from build123d import *

# Parameters (mm, degrees)
EXTRUDE_THIN1_DEPTH = 206.375
FILLET1_R           = 1.27


with BuildPart() as part:
    # Sketch1 → Extrude-Thin1 (new body)
    with BuildSketch(Plane.XY):
        with BuildLine():
            Line((0, 0), (-1.5875, 0))
            Line((-1.5875, 0), (-1.5875, 2.38125))
            ThreePointArc((-1.5875, 2.38125), (-4.95373921, 4.191798454), (-6.35, 7.749902995))
            ThreePointArc((-6.35, 7.749902995), (-7.0533091, 9.486054835), (-8.73125, 10.31875))
            Line((-8.73125, 10.31875), (-8.73125, 11.90625))
            ThreePointArc((-8.73125, 11.90625), (-10.983204711, 13.93861616), (-10.254760064, 16.883303007))
            ThreePointArc((-10.254760064, 16.883303007), (-8.456232552, 18.243920166), (-6.35, 19.05))
            Line((-6.35, 19.05), (-6.35, 20.6375))
            Line((-6.35, 20.6375), (0, 20.6375))
            Line((0, 20.6375), (0, 19.3675))
            Line((0, 19.3675), (-5.08, 19.3675))
            Line((-5.08, 19.3675), (-5.08, 17.961479369))
            ThreePointArc((-5.08, 17.961479369), (-7.394462244, 17.359516713), (-9.353746016, 15.988275809))
            ThreePointArc((-9.353746016, 15.988275809), (-9.540424793, 13.84093001), (-7.46125, 13.272621004))
            Line((-7.46125, 13.272621004), (-7.46125, 11.290352642))
            ThreePointArc((-7.46125, 11.290352642), (-5.752972349, 9.885293584), (-5.080314797, 7.778178184))
            ThreePointArc((-5.080314797, 7.778178184), (-3.615692697, 4.649806034), (-0.3175, 3.623280274))
            Line((-0.3175, 3.623280274), (-0.3175, 1.27))
            Line((-0.3175, 1.27), (0, 1.27))
            Line((0, 1.27), (0, 0))
        make_face()
    extrude(amount=-EXTRUDE_THIN1_DEPTH)

    # Fillet1
    fillet1_edges = [part.edges().sort_by_distance(p)[0] for p in [
        (-5.08, 17.961479369, -103.1875),
        (-7.46125, 13.272621004, -103.1875),
        (-6.35, 20.6375, -103.1875),
    ]]
    fillet(fillet1_edges, radius=FILLET1_R)


solid = part.part
Check sheet for the modelled part. Datum: model origin and axes. Units: mm. A direction names the side the tool comes from. Give positions to 0.01 mm unless a question says otherwise; leave off trailing zeros. Loops run counter-clockwise (first coordinate to the right, second up) from the corner with the lowest first, then second, coordinate; pieces in that order, holes last. Notation, with made-up numbers: M 69.5,71 L 81.5,71 A30 cw 81.5,104 Z; hole C 12,28 d8. An arc over 180 degrees is marked long. Use a Markdown table: item, result. Add a question column.
Q1. Scan lines: line 1 along Y through (x, z) = (-4.75, -111); line 2 along Y through (x, z) = (-0.5, -190.5); line 3 along X through (y, z) = (7.5, -77). Record each from-to range of solid material in increasing order. Write a range as [from, to].
Q2. Sectioned sample at B-B, the plane x = -3.25. Record the cut outline in (y, z) (1 decimal).
Q3. Go/stop test with flat-tipped pins: pin 1 (1.2 mm diameter, centred on y = 1, z = -84.5, fed in from -X); pin 2 (6 mm diameter, centred on y = 9.5, z = -105, fed in from -X); pin 3 (1 mm diameter, centred on y = 9.5, z = -44.5, fed in from +X). Record where each tip stops, or that it passes through.
Q4. Mould release check, pull along Y, two halves, no side actions. Record for faces 1 (the cylindrical face through (-7.817, 17.146, -101.743)), 2 (the flat face through (-6.4, 10.4, -206.375)), 3 (the cylindrical face through (-11, 14, -102)), 4 (the flat face through (-3, 20.638, -102)): pulls with the +Y half, pulls with the -Y half, needs draft (parallel to the pull), parting line crosses it, or undercut.
Q5. Tool access check on faces 5 (the cylindrical face through (-8.48, 18.23, -101.74)), 6 (the flat face through (-3, 19.368, -102)). Record the directions out of +Z, -Z, +X, -X, +Y, -Y that give a thin tool (end or side, any length) a straight path to the whole face; none if there is none.
Q6. Sectioned sample at A-A, the plane z = -132. Record the cut outline in (x, y), then the cut area to 3 significant figures.
Verdict:
| question | item | result |
|---|---|---|
| 1 | line 1 | [3.97, 6.22], [19.37, 20.64] |
| 1 | line 2 | [0, 3.61], [19.37, 20.64] |
| 1 | line 3 | [-6.34, -5.07] |
| 2 | outline | M 2.9,-206.4 L 4.4,-206.4 L 4.4,0 L 2.9,0 Z; M 19.4,-206.4 L 20.6,-206.4 L 20.6,0 L 19.4,0 Z |
| 3 | pin 1 | x = -1.59 |
| 3 | pin 2 | x = -10.01 |
| 3 | pin 3 | x = -5.3 |
| 4 | face 1 | undercut |
| 4 | face 2 | needs draft |
| 4 | face 3 | parting line crosses it |
| 4 | face 4 | pulls with the +Y half |
| 5 | face 5 | +Z, -Z, -X, +Y |
| 5 | face 6 | +Z, -Z, +X |
| 6 | outline | M -10.25,16.88 A2.95 ccw -8.73,11.91 L -8.73,10.32 A2.64 cw -6.35,7.75 A5.55 ccw -1.59,2.38 L -1.59,0 L 0,0 L 0,1.27 L -0.32,1.27 L -0.32,3.62 A4.28 cw -5.08,7.78 A3.91 ccw -7.46,11.29 L -7.46,11.91 A1.27 ccw -8.49,13.15 A1.68 cw -9.35,15.99 A6.75 cw -6.07,17.81 A1.27 ccw -5.08,19.05 L -5.08,19.37 L 0,19.37 L 0,20.64 L -5.08,20.64 A1.27 ccw -6.35,19.37 L -6.35,19.05 A8.02 ccw Z |
| 6 | area | 42.3 mm^2 |
